```python
from build123d import *

# Parameters (mm, degrees)
F0_R     = 1.5875
F1_DEPTH = 4.7625
F3_DEPTH = 58.1406
F5_DEPTH = 69.215
F7_DEPTH = 25.4


with BuildPart() as f1:
    # F0 (on Top) → F1 (new body)
    with BuildSketch(Plane.XY):
        Polygon((-17.145, 87.89836), (-42.545, 87.89836), (-42.545, 0), (-45.72, 0), (-45.72, -58.15164), (-42.545, -58.15164), (-42.545, -66.08914), (-34.6075, -66.08914), (-34.6075, -69.26414), (34.6075, -69.26414), (34.6075, -66.08914), (42.545, -66.08914), (42.545, -58.15164), (45.72, -58.15164), (45.72, 0), (42.545, 0), (42.545, 87.89836), (17.145, 87.89836), (17.145, 27.487862), (12.7, 27.487862), (12.7, 91.07336), (-12.7, 91.07336), (-12.7, 27.487862), (-17.145, 27.487862), align=None)
        with Locations((-31.75, -43.86414)):
            Circle(F0_R, mode=Mode.SUBTRACT)
        with Locations((31.75, -43.86414)):
            Circle(F0_R, mode=Mode.SUBTRACT)
        with Locations((-31.75, 57.73586)):
            Circle(F0_R, mode=Mode.SUBTRACT)
        with Locations((31.75, 57.73586)):
            Circle(F0_R, mode=Mode.SUBTRACT)
    extrude(amount=F1_DEPTH)

    # F2 (on face) → F3 (join)
    with BuildSketch(Plane.XZ.offset(58.15164)):
        with BuildLine():
            Line((-45.72, 20.0025), (-45.72, 4.7625))
            Line((-45.72, 4.7625), (-42.545, 4.7625))
            Line((-42.545, 4.7625), (-42.545, 20.0025))
            ThreePointArc((-42.545, 20.0025), (-42.225108, 20.927946), (-41.402, 21.458299))
            ThreePointArc((-41.402, 21.458299), (-40.126284, 23.045799), (-41.402, 24.633299))
            ThreePointArc((-41.402, 24.633299), (-44.485221, 23.179692), (-45.72, 20.0025))
        make_face()
        with BuildLine():
            Line((42.545, 20.0025), (42.545, 4.7625))
            Line((42.545, 4.7625), (45.72, 4.7625))
            Line((45.72, 4.7625), (45.72, 20.0025))
            ThreePointArc((45.72, 20.0025), (44.485221, 23.179692), (41.402, 24.633299))
            ThreePointArc((41.402, 24.633299), (40.126284, 23.045799), (41.402, 21.458299))
            ThreePointArc((41.402, 21.458299), (42.225108, 20.927946), (42.545, 20.0025))
        make_face()
    extrude(amount=-F3_DEPTH)

    # F4 (on face) → F5 (join)
    with BuildSketch(Plane.YZ.offset(34.6075)):
        with BuildLine():
            Line((-69.26414, 20.0025), (-69.26414, 4.7625))
            Line((-69.26414, 4.7625), (-66.08914, 4.7625))
            Line((-66.08914, 4.7625), (-66.08914, 20.0025))
            ThreePointArc((-66.08914, 20.0025), (-65.769247, 20.927946), (-64.94614, 21.458299))
            ThreePointArc((-64.94614, 21.458299), (-63.670424, 23.045799), (-64.94614, 24.633299))
            ThreePointArc((-64.94614, 24.633299), (-68.029361, 23.179692), (-69.26414, 20.0025))
        make_face()
    extrude(amount=-F5_DEPTH)

    # F6 (on face) → F7 (join)
    with BuildSketch(Plane.YZ.offset(12.7)):
        with BuildLine():
            Line((87.89836, 4.7625), (91.07336, 4.7625))
            Line((91.07336, 4.7625), (91.07336, 9.5377))
            ThreePointArc((91.07336, 9.5377), (89.48586, 11.1252), (87.89836, 9.5377))
            Line((87.89836, 9.5377), (87.89836, 4.7625))
        make_face()
    extrude(amount=-F7_DEPTH)


solid = f1.part
```
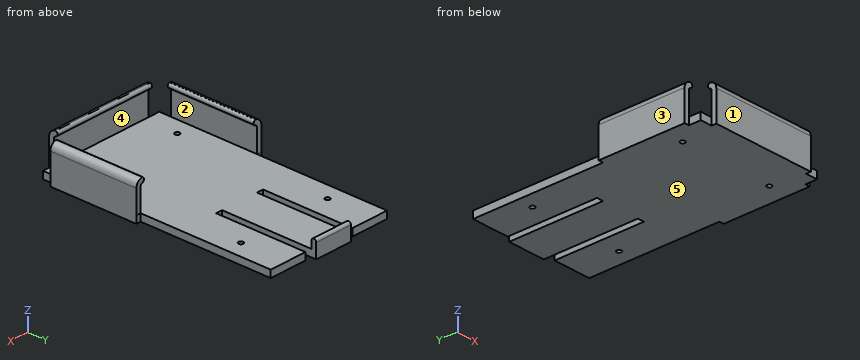
Input: part model. Units: mm. Frame: model coordinates. Face numbers are marked on the shaded views. A direction names the side the tool comes from. Give positions to 0.01 mm unless a question says otherwise; leave off trailing zeros. Order: outer loops, then holes, each group sorted by start corner. A loop starts at its lowest first (then second) coordinate and runs counter-clockwise, first axis right, second up. Notation, with made-up numbers: M -15,74.25 L 10,74.25 A27 ccw 10,105.25 Z; hole C 84,-0.75 d11. An arc over 180 degrees is marked long. Return JSON: item names as keys, results as strings.
Item 1: Ray query, probe 1 along Y at (x, z) = (-31.75, 3.75); probe 2 along X at (y, z) = (-54, 7.75) (3 decimals); probe 3 along Z at (x, y) = (-8.5, 46). Return the intervals inside material, ascending.
Solutions:
{"probe 1": "-69.26 to -45.45, -42.28 to 56.15, 59.32 to 87.9", "probe 2": "-45.72 to -42.545, 42.545 to 45.72", "probe 3": "0 to 4.76"}
Item 2: Pull-direction query (Z, two-part tool) for the marked faces 3, 4 and 5; classes: +Z half, -Z half, draft (parallel to the pull), parting line (faces both ways), or undercut.
Solutions:
{"face 3": "draft", "face 4": "undercut", "face 5": "-Z half"}
Item 3: Cut plane A-A (x = 31.75). Return loops of the section in (y, z).
Solutions:
{"outline": "M -69.26,0 L -45.45,0 L -45.45,4.76 L -66.09,4.76 L -66.09,20 A1.5 cw -64.95,21.46 A1.63 ccw -64.95,24.63 A4.6 ccw -69.26,20 Z; M -42.28,0 L 56.15,0 L 56.15,4.76 L -42.28,4.76 Z; M 59.32,0 L 87.9,0 L 87.9,4.76 L 59.32,4.76 Z"}
Item 4: Access query for the marked faces 1 and 2. Directions: +Z, -Z, +X, -X, +Y, -Y. A direction counts if a zero-diameter tool reaches every point of the face in a straight line with its end or side. Return the directions, or none.
Solutions:
{"face 1": "+Z, -Z, +X, -X, -Y", "face 2": "+Y, -Y"}
Item 5: First-contact query: P1, Ø3, axis at y = -66, z = 7.5, coming from the +X side; P2, Ø2.5, axis at y = -60.5, z = 2, coming from the +X side (3 decimals); P3, Ø4, axis at x = -26, z = 3, coming from the +Y side. Flat tips, straight axial feed; report the tip coordinate or a pass-through.
Solutions:
{"P1": "x = 34.61", "P2": "x = 42.545", "P3": "y = 87.9"}
Item 6: Cut plane C-C (z = 7). Return loops of the section in (x, y) (1 decimal).
Solutions:
{"outline": "M -45.7,-58.2 L -42.5,-58.2 L -42.5,0 L -45.7,0 Z; M -34.6,-69.3 L 34.6,-69.3 L 34.6,-66.1 L -34.6,-66.1 Z; M -12.7,87.9 L 12.7,87.9 L 12.7,91.1 L -12.7,91.1 Z; M 42.5,-58.2 L 45.7,-58.2 L 45.7,0 L 42.5,0 Z"}
Item 7: Cut plane B-B (y = 40.5). Return loops of the section in (x, z) (1 decimal), then the cut area to 3 significant figures.
Solutions:
{"outline": "M -42.5,0 L -17.1,0 L -17.1,4.8 L -42.5,4.8 Z; M -12.7,0 L 12.7,0 L 12.7,4.8 L -12.7,4.8 Z; M 17.1,0 L 42.5,0 L 42.5,4.8 L 17.1,4.8 Z", "area": "363 mm^2"}
Item 8: Cut plane D-D (y = -33.5). Return loops of the section in (x, z) (1 decimal), then the cut area to 3 significant figures.
Solutions:
{"outline": "M -45.7,0 L 45.7,0 L 45.7,20 A4.6 ccw 41.4,24.6 A1.6 ccw 41.4,21.5 A1.5 cw 42.5,20 L 42.5,4.8 L -42.5,4.8 L -42.5,20 A1.5 cw -41.4,21.5 A1.6 ccw -41.4,24.6 A4.6 ccw -45.7,20 Z", "area": "567 mm^2"}
